```python
from build123d import *

# Parameters (mm, degrees)
BOSS_EXTRUDE1_DEPTH = 2.5
SKETCH2_R           = 2
CUT_EXTRUDE1_DEPTH  = 62.335144901


with BuildPart() as part:
    # Sketch1 → Boss-Extrude1 (new, symmetric)
    with BuildSketch(Plane.XY):
        with BuildLine():
            Line((0, 4), (57, 4))
            ThreePointArc((57, 4), (61, 0), (57, -4))
            Line((57, -4), (0, -4))
            ThreePointArc((0, -4), (-4, 0), (0, 4))
        make_face()
    extrude(amount=BOSS_EXTRUDE1_DEPTH, both=True)

    # Sketch2 → Cut-Extrude1 (cut, through all)
    with BuildSketch(Plane.XY.offset(2.5)):
        with Locations((57, 0)):
            Circle(SKETCH2_R)
        Circle(SKETCH2_R)
    extrude(amount=-CUT_EXTRUDE1_DEPTH, mode=Mode.SUBTRACT)


solid = part.part
```
Work out the finished part from the listing and answer in its coordinate system (mm). Coordinates: 2 decimals unless noted, no trailing zeros. Write each loop counter-clockwise with the first axis right and the second up, starting at its lowest first coordinate (ties: lowest second). Pieces come first, ordered by that corner, then holes. Notation, with made-up numbers: (81.25, 4.25) - (140.25, 4.25) arc R4 ccw to (140.25, 10.25) - close; hole circle Ø5 at (13, 3.5). An arc over 180 degrees is marked (long way). Answer as a JSON object with one key per item and string values.
Q1. Consider L1, parallel to X at y = 1, z = -1.85; L2, parallel to X at y = -1.5, z = -0.2; L3, parallel to Y at x = 57, z = -0.2. Determine where each line is inside the solid, lowest interval first. Write a range as from..to.
Results list:
{"L1": "x = -3.87..-1.73, 1.73..55.27, 58.73..60.87", "L2": "x = -3.71..-1.32, 1.32..55.68, 58.32..60.71", "L3": "y = -4..-2, 2..4"}
Q2. For a pull along X with two mould halves and no side action, classify faces 1 (the cylindrical face through (0, -2, 0)), 2 (the cylindrical face through (61, 0, 0)), 3 (the cylindrical face through (-4, 0, 0)) as pulls with the +X half, pulls with the -X half, needs draft (parallel to the pull), parting line crosses it, or undercut.
Results list:
{"face 1": "undercut", "face 2": "pulls with the +X half", "face 3": "pulls with the -X half"}
Q3. Find section A-A (y = 0). Write down the section's boundary in (x, z), plus the area to 3 significant figures.
Results list:
{"outline": "(-4, -2.5) - (-2, -2.5) - (-2, 2.5) - (-4, 2.5) - close; (2, -2.5) - (55, -2.5) - (55, 2.5) - (2, 2.5) - close; (59, -2.5) - (61, -2.5) - (61, 2.5) - (59, 2.5) - close", "area": "285 mm^2"}
Q4. Find section B-B (z = 1.1). Write down the section's boundary in (x, y).
Results list:
{"outline": "(0, -4) - (57, -4) arc R4 ccw to (57, 4) - (0, 4) arc R4 ccw to start; hole circle Ø4 at (0, 0); hole circle Ø4 at (57, 0)"}
Q5. Given pin 1 Ø1 at (y, z) = (1.5, 0) entering from -X; pin 2 Ø1 at (y, z) = (1.5, -1.5) entering from +X, each flat-ended and moving along its own axis, determine where each tip first touches the part or whether it passes through.
Results list:
{"pin 1": "stops at x = -3.87", "pin 2": "stops at x = 60.87"}
